Autodesk Inventor part; units mm, degrees
ref_plane "YZ Plane" through (0, 0, 0) normal (1, 0, 0) x (0, 1, 0)
ref_plane "XZ Plane" through (0, 0, 0) normal (0, 1, 0) x (-1, 0, 0)
ref_plane "XY Plane" through (0, 0, 0) normal (0, 0, 1) x (1, 0, 0)
sketch "Эскиз2" plane through (0, 0, 0) normal (0, 0, 1) x (1, 0, 0)
  line L0 (-4.9, 3) -> (-4.9, 1.6)
  line L1 (-4.9, 1.6) -> (-3.3, 0)
  line L2 (-3.3, 0) -> (0, 0)
  line L3 (-4.9, 3) -> (-2.9, 3)
  line L4 (-2.9, 3) -> (-2.9, 5)
  line L5 (-2.9, 5) -> (0, 5)
  line L6 (-6.86, 0) -> (6.86, 0)
  line L7 (0, -1) -> (0, 6)
  line L8 (4.9, 3) -> (4.9, 1.6)
  line L9 (4.9, 1.6) -> (3.3, 0)
  line L10 (3.3, 0) -> (0, 0)
  line L11 (4.9, 3) -> (2.9, 3)
  line L12 (2.9, 3) -> (2.9, 5)
  line L13 (2.9, 5) -> (0, 5)
  point P0 (3.3, 0)
  dimension "d0" = 2
  dimension "d1" = 1.4
  dimension "d3" = 9.8
  dimension "d4" = 5.8
  dimension "d5" = 5
  dimension "d18" = 6.6
extrude "Выдавливание1" add sketch "Эскиз2" along normal mid plane 10
sketch "Эскиз3" plane through (-2.9, 5, 5) normal (0, 1, 0) x (1, 0, 0)
  point P0 (2.9, 5)
  point P1 (2.9, 5)
hole "Отверстие1" at (0, 5, 0) direction (0, -1, 0) diameter 4.134 end through all
properties part number "гайка T-паза m6"
Model file for the job. Use its own axes, mm. A direction names the side the tool comes from. Give positions to 0.01 mm unless a question says otherwise; leave off trailing zeros. Write each loop counter-clockwise with the first axis right and the second up, starting at its lowest first coordinate (ties: lowest second). Pieces come first, ordered by that corner, then holes. Notation, with made-up numbers: (60, 28) -> (99, 28) arc R22 cw to (99, 60) -> close; hole circle Ø2 at (87, 85). An arc over 180 degrees is marked (long way). Write item = value, one per line.
(1) Slice it at A-A, the plane x = 0. Give the cut face in (y, z).
Determined:
outline = (0, -5) -> (5, -5) -> (5, -2.07) -> (0, -2.07) -> close; (0, 2.07) -> (5, 2.07) -> (5, 5) -> (0, 5) -> close
(2) Probe line 1 along Z through (x, y) = (0, 0.3); line 2 along X through (y, z) = (2.95, 0); line 3 along Y through (x, z) = (3, -0.75). List the from-to ranges inside material, lowest first.
Determined:
line_1 = -5 to -2.07, 2.07 to 5
line_2 = -4.9 to -2.07, 2.07 to 4.9
line_3 = 0 to 3
(3) Flat gauge pins, fed straight in: P1, Ø1, axis at y = 4.5, z = 1, coming from the +X side; P2, Ø1, axis at y = 4, z = -0.5, coming from the -X side; P3, Ø1, axis at x = -2.5, z = -1, coming from the -Y side; P4, Ø1, axis at x = -3.5, z = 0, coming from the +Y side. Where does each tip first touch, or does it go through?
Determined:
P1 = 2.9
P2 = -2.9
P3 = 0
P4 = 3
(4) Mould opens along Y. For faces 3 (the face through (-2.25, 0, -0.07)), 4 (the face through (-2.9, 4, 0)), 5 (the face through (-4, 3, 0)) say: released by +Y, released by -Y, zero draft, split by the parting line, or undercut.
Determined:
face_3 = released by -Y
face_4 = zero draft
face_5 = released by +Y
(5) Slice it at D-D, the plane z = 3.25. Give the cut face in (x, y), then the cut area to 3 significant figures.
Determined:
outline = (-4.9, 1.6) -> (-3.3, 0) -> (3.3, 0) -> (4.9, 1.6) -> (4.9, 3) -> (2.9, 3) -> (2.9, 5) -> (-2.9, 5) -> (-2.9, 3) -> (-4.9, 3) -> close
area = 38.4 mm2
(6) Slice it at B-B, the plane z = 0. Give the cut face in (x, y).
Determined:
outline = (-4.9, 1.6) -> (-3.3, 0) -> (-2.07, 0) -> (-2.07, 5) -> (-2.9, 5) -> (-2.9, 3) -> (-4.9, 3) -> close; (2.07, 0) -> (3.3, 0) -> (4.9, 1.6) -> (4.9, 3) -> (2.9, 3) -> (2.9, 5) -> (2.07, 5) -> close
(7) Slice it at C-C, the plane y = 4.7. Give the cut face in (x, z).
Determined:
outline = (-2.9, -5) -> (2.9, -5) -> (2.9, 5) -> (-2.9, 5) -> close; hole circle Ø4.13 at (0, 0)
(8) Tool access for faces 1 (the face through (2.9, 4, 0)), 2 (the face through (0, 5, -2.3)): list every direction of +Z, -Z, +X, -X, +Y, -Y with a clear straight run to the whole face (end or side of a thin tool).
Determined:
face_1 = +Z, -Z, +X, +Y
face_2 = +Z, -Z, +X, -X, +Y
